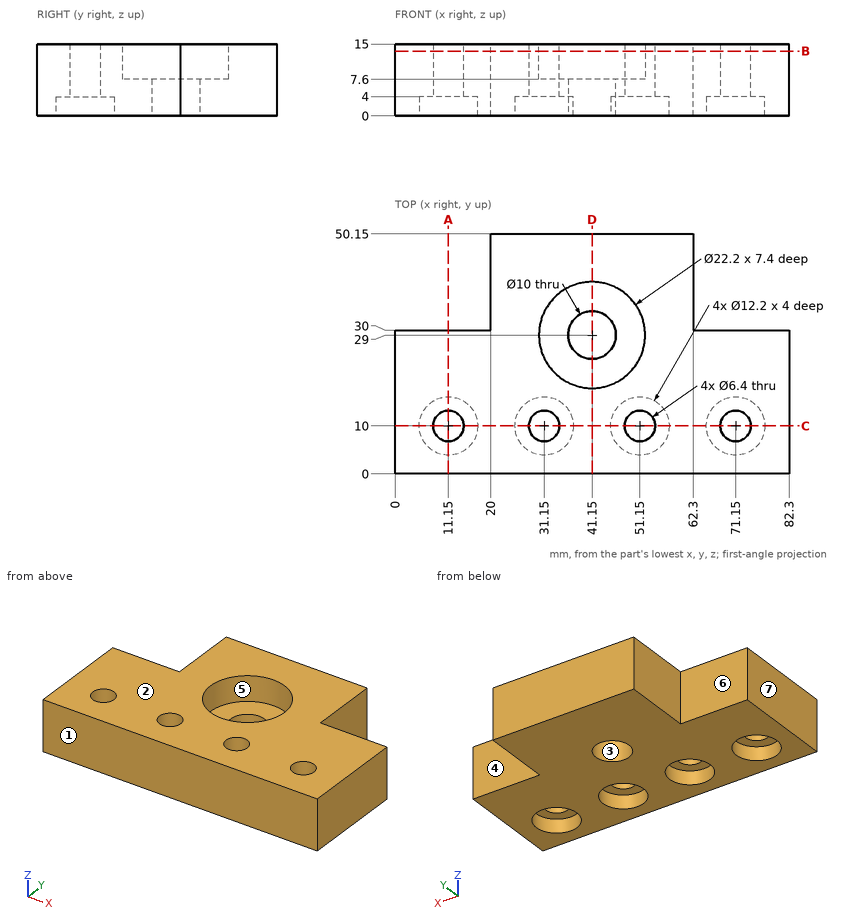
The figure shows three views and two pictorial views of one solid part (mm, origin at its lowest corner). Answer the questions. A direction names the side the tool comes from. Round coordinates to 2 decimals unless told otherwise and drop trailing zeros. Order: outer loops, then holes, each group sorted by start corner. A loop starts at its lowest first (then second) coordinate and runs counter-clockwise, first axis right, second up. Notation, with made-up numbers: M -12,-39.5 L 30,-39.5 A34 ccw 30,-1.5 Z; hole C -19.5,-3 d4. An arc over 180 degrees is marked long. Put each result on its own line as item: value. Start each with the question number.
Q1. Flat-ended cylindrical pins translate along their axes: pin 1 (19.5 mm diameter, centred on x = 51.15, y = 10, fed in from -Z); pin 2 (6.5 mm diameter, centred on x = 45.5, y = 26.5, fed in from +Z); pin 3 (10 mm diameter, centred on x = 31.15, y = 10, fed in from -Z); pin 4 (4.5 mm diameter, centred on x = 77, z = 9, fed in from +Y). Find the tip coordinate at first contact, or state that the pin passes through.
Q2. Section A-A, the plane x = 11.15 is taken. Write down the section's boundary in (y, z), and give its area (3 significant figures).
Q3. For a pull along Y with two mould halves and no side action, classify the marked faces 1, 2 and 3 as pulls with the +Y half, pulls with the -Y half, needs draft (parallel to the pull), parting line crosses it, or undercut.
Q4. Section B-B, the plane z = 13.5 is taken. Write down the section's boundary in (x, y).
Q5. Straight lines are drawn through the part: L1, parallel to X at y = 10, z = 8.75; L2, parallel to Y at x = 11.15, z = 7.5; L3, parallel to Y at x = 11.15, z = 1.45. For each, find the intervals that lie inside material, in ascending order. Write a range as [from, to].
Q6. A tool of negligible diameter and unlimited length cuts with its end or side. For the marked faces 4, 5, 6 and 7, from which of +Z, -Z, +X, -X, +Y, -Y can it reach the whole face along a straight path? Write none if from no direction.
Q7. Section D-D, the plane x = 41.15 is taken. Write down the section's boundary in (y, z), and give its area (3 significant figures).
Q8. Section C-C, the plane y = 10 is taken. Give the number of separate pieces and of enclosed holes in the cut face, and give its area (3 significant figures).
Findings below:
1. pin 1: stops at z = 0
1. pin 2: stops at z = 7.6
1. pin 3: stops at z = 4
1. pin 4: stops at y = 30
2. outline: M 0,0 L 3.9,0 L 3.9,4 L 6.8,4 L 6.8,15 L 0,15 Z; M 13.2,4 L 16.1,4 L 16.1,0 L 30,0 L 30,15 L 13.2,15 Z
2. area: 331 mm^2
3. face 1: pulls with the -Y half
3. face 2: needs draft
3. face 3: undercut
4. outline: M 0,0 L 82.3,0 L 82.3,30 L 62.3,30 L 62.3,50.15 L 20,50.15 L 20,30 L 0,30 Z; hole C 11.15,10 d6.4; hole C 31.15,10 d6.4; hole C 41.15,29 d22.2; hole C 51.15,10 d6.4; hole C 71.15,10 d6.4
5. L1: x = [0, 7.95], [14.35, 27.95], [34.35, 47.95], [54.35, 67.95], [74.35, 82.3]
5. L2: y = [0, 6.8], [13.2, 30]
5. L3: y = [0, 3.9], [16.1, 30]
6. face 4: +Z, -Z, +X, +Y
6. face 5: +Z
6. face 6: +Z, -Z, -X, +Y
6. face 7: +Z, -Z, -X, +Y, -Y
7. outline: M 0,0 L 24,0 L 24,7.6 L 17.9,7.6 L 17.9,15 L 0,15 Z; M 34,0 L 50.15,0 L 50.15,15 L 40.1,15 L 40.1,7.6 L 34,7.6 Z
7. area: 512 mm^2
8. separate pieces: 5
8. enclosed holes: 0
8. area: 758 mm^2
